Design review of the part built by this model. Coordinates are the model's own, in mm. A direction names the side the tool comes from. Give positions to 0.01 mm unless a question says otherwise; leave off trailing zeros. Write each loop counter-clockwise with the first axis right and the second up, starting at its lowest first coordinate (ties: lowest second). Pieces come first, ordered by that corner, then holes. Notation, with made-up numbers: (36.25, 43) - (80.25, 43) arc R17 cw to (80.25, 62) - close; hole circle Ø11 at (27, 7). An arc over 180 degrees is marked (long way). Use a Markdown table: item, result. Add a question column.
```python
from build123d import *

# Parameters (mm, degrees)
SKETCH1_W           = 80
SKETCH1_H           = 50
BOSS_EXTRUDE1_DEPTH = 5
SKETCH2_R           = 3.6
CUT_EXTRUDE1_DEPTH  = 123.886126149
SKETCH3_R           = 1.5
CUT_EXTRUDE2_DEPTH  = 123.886126149
SKETCH4_R           = 11.1
CUT_EXTRUDE3_DEPTH  = 2
SKETCH5_R           = 11
CUT_EXTRUDE4_DEPTH  = 123.886126149
SKETCH7_W           = 80
SKETCH7_H           = 30
BOSS_EXTRUDE2_DEPTH = 5
SKETCH13_W          = 80
SKETCH13_H          = 5
BOSS_EXTRUDE3_DEPTH = 50
CUT_EXTRUDE6_REACH  = 129.519
SKETCH14_R          = 15
CUT_EXTRUDE7_REACH  = 129.519
SKETCH16_R          = 1.75
CHAMFER1_SIZE       = 10


with BuildPart() as part:
    # Sketch1 → Boss-Extrude1 (new body)
    with BuildSketch(Plane.XY):
        with Locations((-80, -1)):
            Rectangle(SKETCH1_W, SKETCH1_H)
    extrude(amount=BOSS_EXTRUDE1_DEPTH)

    # Sketch2 → Cut-Extrude1 (cut, through all)
    with BuildSketch(Plane.XY.offset(5)):
        with Locations((-100, -1)):
            Circle(SKETCH2_R)
    extrude(amount=-CUT_EXTRUDE1_DEPTH, mode=Mode.SUBTRACT)

    # Sketch3 → Cut-Extrude2 (cut, through all)
    with BuildSketch(Plane.XY.offset(5)):
        with Locations((-91.25, -1)):
            Circle(SKETCH3_R)
        with Locations((-108.75, -1)):
            Circle(SKETCH3_R)
    extrude(amount=-CUT_EXTRUDE2_DEPTH, mode=Mode.SUBTRACT)

    # Sketch4 → Cut-Extrude3 (cut)
    with BuildSketch(Plane.XY.offset(5)):
        with Locations((-100, -1)):
            Circle(SKETCH4_R)
    extrude(amount=-CUT_EXTRUDE3_DEPTH, mode=Mode.SUBTRACT)

    # Sketch5 → Cut-Extrude4 (cut, through all)
    with BuildSketch(Plane.XY.offset(5)):
        with Locations((-59.5, -1)):
            Circle(SKETCH5_R)
    cut_extrude4 = extrude(amount=-CUT_EXTRUDE4_DEPTH, mode=Mode.SUBTRACT)

    # Sketch7 → Boss-Extrude2 (add)
    with BuildSketch(Plane.XZ.offset(26)):
        with Locations((-80, -10)):
            Rectangle(SKETCH7_W, SKETCH7_H)
    extrude(amount=BOSS_EXTRUDE2_DEPTH)

    # Sketch13 → Boss-Extrude3 (add)
    with BuildSketch(Plane(origin=(0, -26, 0), x_dir=(1, 0, 0), z_dir=(0, 1, 0))):
        with Locations((-80, 22.5)):
            Rectangle(SKETCH13_W, SKETCH13_H)
    extrude(amount=BOSS_EXTRUDE3_DEPTH)

    # Sketch14 → Cut-Extrude6 (cut, up to next)
    with BuildSketch(Plane(origin=(0, 0, -25), x_dir=(-1, 0, 0), z_dir=(0, 0, -1)), mode=Mode.PRIVATE) as cut_extrude6_sk1:
        with Locations((100, -1)):
            Circle(SKETCH14_R)
    cut_extrude6_tool1 = extrude(cut_extrude6_sk1.sketch, amount=-CUT_EXTRUDE6_REACH, mode=Mode.PRIVATE) & part.part
    add(cut_extrude6_tool1.solids().sort_by_distance((-100, -1, -25))[0], mode=Mode.SUBTRACT)

    # Sketch16 → Cut-Extrude7 (cut, up to next)
    with BuildSketch(Plane(origin=(0, 0, -25), x_dir=(-1, 0, 0), z_dir=(0, 0, -1)), mode=Mode.PRIVATE) as cut_extrude7_sk1:
        with Locations((83.382990642, 15.617009358)):
            Circle(SKETCH16_R)
    cut_extrude7_tool1 = extrude(cut_extrude7_sk1.sketch, amount=-CUT_EXTRUDE7_REACH, mode=Mode.PRIVATE) & part.part
    # Sketch16 → Cut-Extrude7 (cut, up to next)
    with BuildSketch(Plane(origin=(0, 0, -25), x_dir=(-1, 0, 0), z_dir=(0, 0, -1)), mode=Mode.PRIVATE) as cut_extrude7_sk2:
        with Locations((116.617009358, -17.617009358)):
            Circle(SKETCH16_R)
    cut_extrude7_tool2 = extrude(cut_extrude7_sk2.sketch, amount=-CUT_EXTRUDE7_REACH, mode=Mode.PRIVATE) & part.part
    add(cut_extrude7_tool1.solids().sort_by_distance((-83.382991, 15.617009, -25))[0], mode=Mode.SUBTRACT)
    add(cut_extrude7_tool2.solids().sort_by_distance((-116.617009, -17.617009, -25))[0], mode=Mode.SUBTRACT)

    # Mirror6: Cut-Extrude4 across plane
    add(cut_extrude4.mirror(Plane(origin=(0, 0, -10), x_dir=(1, 0, 0), z_dir=(0, 0, -1))), mode=Mode.SUBTRACT)

    # Chamfer1
    chamfer1_edges = [part.edges().sort_by_distance(p)[0] for p in [
        (-40, 24, -22.5),
        (-120, 24, -22.5),
        (-120, 24, 2.5),
        (-40, 24, 2.5),
    ]]
    chamfer(chamfer1_edges, length=CHAMFER1_SIZE)


solid = part.part
```
(1) For line 1 along Z through (x, y) = (-109.5, -14); line 2 along X through (y, z) = (3.5, -22); line 3 along Y through (x, z) = (-59.5, -22.6), list the stretches that pass through material, from the lowest coordinate up.
(2) Add section A-A (y = 19.5). State the section outline as (x, z) points.
(3) Tool access review of faces 5 (the face through (-103, 2, 3)), 6 (the face through (-114.307, 3.506, -22.535)), 7 (the face through (-81, -1, -20)): name each direction out of +Z, -Z, +X, -X, +Y, -Y from which nothing blocks a thin tool from reaching the whole face with its end or side.
(4) Add section D-D (y = -1). Count the separate pieces of the cut face and the enclosed holes in it, and give its area (3 significant figures).
(5) Mouldability with a two-part tool opening along Z and no side actions: class faces 1 (the face through (-81, -1, 0)), 2 (the face through (-81, -4, -25)), 3 (the face through (-81, -26, -10)), 4 (the face through (-118.234, -18.287, -22.535)) as +Z half, -Z half, draft (parallel to the pull), parting line (faces both ways), or undercut.
(6) Insertion check: pin 1 (1.5 mm diameter, centred on x = -55.5, z = -8, fed in from +Y); pin 2 (8.5 mm diameter, centred on x = -100, y = -1, fed in from +Z); pin 3 (3.5 mm diameter, centred on x = -91.25, y = -1, fed in from -Z). Each pin has a flat end and moves straight along its axis. Give the tip position at first contact, or say it passes through.
(7) Add section B-B (x = -59.5). State the section outline as (y, z) points, and give its area (3 significant figures).
(8) Add section C-C (x = -47). State the section outline as (y, z) points.
Answers follow:
| question | item | result |
|---|---|---|
| 1 | line 1 | -25 to -20, 0 to 5 |
| 1 | line 2 | -120 to -114.31, -85.69 to -69.54, -49.46 to -40 |
| 1 | line 3 | -31 to -12, 10 to 24 |
| 2 | outline | (-114.5, -25) - (-45.5, -25) - (-45.5, -20) - (-114.5, -20) - close; (-114.5, 0) - (-45.5, 0) - (-45.5, 5) - (-114.5, 5) - close |
| 3 | face 5 | +Z |
| 3 | face 6 | -Z |
| 3 | face 7 | +X, -X, +Y |
| 4 | separate pieces | 8 |
| 4 | enclosed holes | 0 |
| 4 | area | 346 mm^2 |
| 5 | face 1 | undercut |
| 5 | face 2 | -Z half |
| 5 | face 3 | undercut |
| 5 | face 4 | draft |
| 6 | pin 1 | y = -26 |
| 6 | pin 2 | z = 3 |
| 6 | pin 3 | z = 0 |
| 7 | outline | (-31, -25) - (-12, -25) - (-12, -20) - (-26, -20) - (-26, 0) - (-12, 0) - (-12, 5) - (-31, 5) - close; (10, -25) - (24, -25) - (24, -20) - (10, -20) - close; (10, 0) - (24, 0) - (24, 5) - (10, 5) - close |
| 7 | area | 430 mm^2 |
| 8 | outline | (-31, -25) - (21, -25) - (21, -20) - (-26, -20) - (-26, 0) - (21, 0) - (21, 5) - (-31, 5) - close |
